Model file for the job. Use its own axes, mm. Face numbers are marked on the shaded views. A direction names the side the tool comes from. Coordinates: 2 decimals unless noted, no trailing zeros. Order: outer loops, then holes, each group sorted by start corner. A loop starts at its lowest first (then second) coordinate and runs counter-clockwise, first axis right, second up. Notation, with made-up numbers: (-9.5, -1) -> (34.5, -1) arc R16 cw to (34.5, 9) -> close; hole circle Ø10 at (-14.5, -2). An arc over 180 degrees is marked (long way). Write item = value, one per line. Start each with the question number.
Q1. Cut at A-A, the plane y = 34. List the corners of the cut face in (x, z), plus the area to 3 significant figures.
Q2. Cut at C-C, the plane x = -14.25. Give the number of separate pieces and of enclosed holes in the cut face, plus the area to 3 significant figures.
Q3. Mould opens along X. For the marked faces 1, 2 and 3 say: +X half, -X half, draft (parallel to the pull), parting line (faces both ways), or undercut.
Q4. Flat gauge pins, fed straight in: pin 1 (6 mm diameter, centred on x = -1, y = 22.5, fed in from -Z); pin 2 (2.5 mm diameter, centred on x = 1, z = 11, fed in from +Y); pin 3 (1.2 mm diameter, centred on x = 2.5, z = 11, fed in from +Y); pin 4 (5 mm diameter, centred on x = 2.5, z = 8, fed in from -Y). Where does each tip first touch, or does it go through?
Q5. 3-axis set-ups, long thin cutter, end or side, ignore diameter. For the marked faces 4, 5, 6 and 7: which of +Z, -Z, +X, -X, +Y, -Y reach the whole face in a straight line?
Q6. Cut at B-B, the plane z = -15. List the corners of the cut face in (x, y), plus the area to 3 significant figures.
Q7. Wall check: line 1 (X direction, y = 37.05, z = 0); line 2 (X direction, y = 35, z = 0); line 3 (Z direction, x = 14.25, y = 1.5) (3 decimals). Give the ranges that are in metal, low to high. Write a range as from..to.
from build123d import *

# Parameters (mm, degrees)
SKETCH1_W               = 48
SKETCH1_H               = 20
BOSS_EXTRUDE1_DEPTH     = 14.5
FILLET1_R               = 1
SKETCH2_R               = 9.5
BOSS_EXTRUDE2_DEPTH     = 25
SKETCH3_W               = 10.545517328
SKETCH3_H               = 9.5
BOSS_EXTRUDE3_DEPTH     = 22
FILLET2_R               = 5
SKETCH4_R               = 1
CUT_EXTRUDE1_DEPTH      = 5
SKETCH5_R               = 7.25
CUT_EXTRUDE2_DEPTH      = 13
SKETCH6_W               = 0.5
SKETCH6_H               = 2
SKETCH8_R               = 7.25
CUT_EXTRUDE3_DEPTH      = 3
SKETCH9_W               = 0.5
SKETCH9_H               = 2
SKETCH11_W              = 9
SKETCH11_H              = 3.5
BOSS_EXTRUDE4_DEPTH     = 3
SKETCH12_W              = 6.5
SKETCH12_H              = 0.5
BOSS_EXTRUDE5_DEPTH     = 0.8
SKETCH13_W              = 9
SKETCH13_H              = 0.25
BOSS_EXTRUDE6_DEPTH     = 1
SKETCH14_W              = 12
SKETCH14_H              = 1.5
BOSS_EXTRUDE7_DEPTH     = 0.8
CUT_EXTRUDE4_DEPTH      = 5
SKETCH16_W              = 7.75
SKETCH16_H              = 7.75
SKETCH16_R              = 2
BOSS_EXTRUDE8_DEPTH     = 2.5
MIRROR4_COPY_1_SKETCH_W = 7.75
MIRROR4_COPY_1_SKETCH_H = 7.75
MIRROR4_COPY_1_SKETCH_R = 2
MIRROR4_COPY_1_DEPTH    = 2.5
FILLET3_RADIUS          = 3.875
FILLET3_LENGTH          = 2.5
FILLET5_RADIUS          = 3.875
FILLET5_LENGTH          = 2.5
FILLET6_RADIUS          = 3.875
FILLET6_LENGTH          = 2.5
FILLET7_RADIUS          = 3.875
FILLET7_LENGTH          = 2.5
FILLET4_R               = 3
SKETCH17_W              = 7
SKETCH17_H              = 1.5
CUT_EXTRUDE5_DEPTH      = 3
SKETCH18_W              = 0.1
SKETCH18_H              = 1.5
BOSS_EXTRUDE9_DEPTH     = 3
SKETCH19_R              = 0.375
BOSS_EXTRUDE10_DEPTH    = 10


with BuildPart() as part:
    # Sketch1 → Boss-Extrude1 (new body)
    with BuildSketch(Plane(origin=(0, 0, 0), x_dir=(1, 0, 0), z_dir=(0, 1, 0))):
        Rectangle(SKETCH1_W, SKETCH1_H)
    extrude(amount=BOSS_EXTRUDE1_DEPTH)

    # Fillet1
    fillet1_edges = [part.edges().sort_by_distance(p)[0] for p in [
        (-24, 7.25, -10),
        (24, 7.25, -10),
        (24, 7.25, 10),
        (-24, 7.25, 10),
    ]]
    fillet(fillet1_edges, radius=FILLET1_R)

    # Sketch2 → Boss-Extrude2 (add)
    with BuildSketch(Plane(origin=(0, 14.5, 0), x_dir=(1, 0, 0), z_dir=(0, 1, 0))):
        with Locations(Location((-13.5, 0, 0), (0, 0, 270))):
            Circle(SKETCH2_R)
        with Locations(Location((13.5, 0, 0), (0, 0, 90))):
            Circle(SKETCH2_R)
    extrude(amount=BOSS_EXTRUDE2_DEPTH)

    # Sketch3 → Boss-Extrude3 (add)
    with BuildSketch(Plane(origin=(0, 14.5, 0), x_dir=(1, 0, 0), z_dir=(0, 1, 0))):
        Rectangle(SKETCH3_W, SKETCH3_H)
    extrude(amount=BOSS_EXTRUDE3_DEPTH)

    # Fillet2
    fillet2_edges = [part.edges().sort_by_distance(p)[0] for p in [
        (-5.272758664, 25.5, -4.75),
        (-5.272758664, 25.5, 4.75),
        (5.272758664, 25.5, 4.75),
        (5.272758664, 25.5, -4.75),
    ]]
    fillet(fillet2_edges, radius=FILLET2_R)

    # Sketch4 → Cut-Extrude1 (cut)
    with BuildSketch(Plane(origin=(0, 36.5, 0), x_dir=(1, 0, 0), z_dir=(0, 1, 0))):
        with Locations(Location((0, 0, 0), (0, 0, 270))):
            Circle(SKETCH4_R)
    extrude(amount=-CUT_EXTRUDE1_DEPTH, mode=Mode.SUBTRACT)

    # Sketch5 → Cut-Extrude2 (cut)
    with BuildSketch(Plane(origin=(0, 39.5, 0), x_dir=(1, 0, 0), z_dir=(0, 1, 0))):
        with Locations(Location((-13.5, 0, 0), (0, 0, 270))):
            Circle(SKETCH5_R)
    extrude(amount=-CUT_EXTRUDE2_DEPTH, mode=Mode.SUBTRACT)

    # Sketch6 → Revolve1 (revolve)
    with BuildSketch(Plane.XY, mode=Mode.PRIVATE) as revolve1_sk:
        with Locations((-20.5, 27.5)):
            Rectangle(SKETCH6_W, SKETCH6_H)
    revolve(revolve1_sk.sketch.rotate(Axis((-13.5, 39.5, 0), (0, -1, 0)), 270), axis=Axis((-13.5, 39.5, 0), (0, -1, 0)))

    # Sketch7 → Revolve2 (revolve)
    with BuildSketch(Plane.XY, mode=Mode.PRIVATE) as revolve2_sk:
        with BuildLine():
            Line((-20.25, 26.5), (-13.5, 26.5))
            Line((-13.5, 26.5), (-13.5, 28.5))
            add(Edge.make_bspline(
                [(-13.5, 28.5), (-20.25, 28.5), (-20.25, 26.5)],
                knots=[4.71238898, 4.71238898, 4.71238898, 6.283185307, 6.283185307, 6.283185307], degree=2, weights=[1, 0.707106781, 1]))
        make_face()
    revolve(revolve2_sk.sketch.rotate(Axis((-13.5, 26.5, 0), (0, 1, 0)), 222.253636979), axis=Axis((-13.5, 26.5, 0), (0, 1, 0)))

    # Sketch8 → Cut-Extrude3 (cut)
    with BuildSketch(Plane(origin=(0, 39.5, 0), x_dir=(1, 0, 0), z_dir=(0, 1, 0))):
        with Locations(Location((13.5, 0, 0), (0, 0, 270))):
            Circle(SKETCH8_R)
    extrude(amount=-CUT_EXTRUDE3_DEPTH, mode=Mode.SUBTRACT)

    # Sketch9 → Revolve3 (revolve)
    with BuildSketch(Plane.XY, mode=Mode.PRIVATE) as revolve3_sk:
        with Locations((20.5, 37.5)):
            Rectangle(SKETCH9_W, SKETCH9_H)
    revolve(revolve3_sk.sketch.rotate(Axis((13.5, 36.5, 0), (0, 1, 0)), 270), axis=Axis((13.5, 36.5, 0), (0, 1, 0)))

    # Sketch11 → Boss-Extrude4 (add)
    with BuildSketch(Plane.XY.offset(10)):
        with Locations((1.5, 9.25)):
            Rectangle(SKETCH11_W, SKETCH11_H)
    extrude(amount=BOSS_EXTRUDE4_DEPTH)

    # Sketch12 → Boss-Extrude5 (add)
    with BuildSketch(Plane.XY.offset(13)):
        with Locations((1.5, 11.25)):
            Rectangle(SKETCH12_W, SKETCH12_H)
    extrude(amount=-BOSS_EXTRUDE5_DEPTH)

    # Sketch13 → Boss-Extrude6 (add)
    with BuildSketch(Plane.XY.offset(13)):
        with Locations((1.5, 7.375)):
            Rectangle(SKETCH13_W, SKETCH13_H)
    extrude(amount=-BOSS_EXTRUDE6_DEPTH)

    # Sketch14 → Boss-Extrude7 (add)
    with BuildSketch(Plane.XY.offset(10)):
        with Locations((1.5, 6.25)):
            Rectangle(SKETCH14_W, SKETCH14_H)
    extrude(amount=BOSS_EXTRUDE7_DEPTH)

    # Sketch15 → Cut-Extrude4 (cut)
    with BuildSketch(Plane.XY.offset(10)):
        Polygon((-4.5, 7), (-4.5, 13), (7.5, 13), (7.5, 7), (6.5, 7), (6.5, 11.5), (-3.5, 11.5), (-3.5, 7), align=None)
    extrude(amount=-CUT_EXTRUDE4_DEPTH, mode=Mode.SUBTRACT)

    # Sketch16 → Boss-Extrude8 (add)
    with BuildSketch(Plane.XZ):
        with Locations((-14.25, 13.875)):
            Rectangle(SKETCH16_W, SKETCH16_H)
        with Locations(Location((-14.25, 13.875, 0), (0, 0, 270))):
            Circle(SKETCH16_R, mode=Mode.SUBTRACT)
    boss_extrude8 = extrude(amount=-BOSS_EXTRUDE8_DEPTH)

    # Mirror3: Boss-Extrude8 across plane
    add(boss_extrude8.mirror(Plane.XY))

    # Mirror4: Boss-Extrude8 across plane
    add(boss_extrude8.mirror(Plane(origin=(0, 0, 0), x_dir=(0, 0, 1), z_dir=(1, 0, 0))))

    # Mirror4 copy 1 sketch → Mirror4 copy 1 (add)
    with BuildSketch(Plane(origin=(0, 0, 0), x_dir=(-1, 0, 0), z_dir=(0, -1, 0))):
        with Locations((-14.25, 13.875)):
            Rectangle(MIRROR4_COPY_1_SKETCH_W, MIRROR4_COPY_1_SKETCH_H)
        with Locations(Location((-14.25, 13.875, 0), (0, 0, 270))):
            Circle(MIRROR4_COPY_1_SKETCH_R, mode=Mode.SUBTRACT)
    extrude(amount=-MIRROR4_COPY_1_DEPTH)

    # Fillet3: full round fillet: the end face becomes a half cylinder, R = half its width
    fillet3_face = Plane((-14.25, 1.25, 17.75), x_dir=(0, -1, 0), z_dir=(0, 0, 1))  # on the end face: x along it, z out of the body
    fillet3_slab = fillet3_face.offset(-FILLET3_RADIUS / 2) * Box(FILLET3_LENGTH, 2 * FILLET3_RADIUS, FILLET3_RADIUS, mode=Mode.PRIVATE)  # the body's end, R deep
    fillet3_round = Plane((-14.25, 1.25, 13.875), x_dir=(0, 0, 1), z_dir=(0, -1, 0)) * Cylinder(FILLET3_RADIUS, FILLET3_LENGTH, mode=Mode.PRIVATE)  # its axis R under the face
    add(fillet3_slab - fillet3_round, mode=Mode.SUBTRACT)

    # Fillet5: full round fillet: the end face becomes a half cylinder, R = half its width
    fillet5_face = Plane((14.25, 1.25, 17.75), x_dir=(0, 1, 0), z_dir=(0, 0, 1))  # on the end face: x along it, z out of the body
    fillet5_slab = fillet5_face.offset(-FILLET5_RADIUS / 2) * Box(FILLET5_LENGTH, 2 * FILLET5_RADIUS, FILLET5_RADIUS, mode=Mode.PRIVATE)  # the body's end, R deep
    fillet5_round = Plane((14.25, 1.25, 13.875), x_dir=(0, 0, 1), z_dir=(0, 1, 0)) * Cylinder(FILLET5_RADIUS, FILLET5_LENGTH, mode=Mode.PRIVATE)  # its axis R under the face
    add(fillet5_slab - fillet5_round, mode=Mode.SUBTRACT)

    # Fillet6: full round fillet: the end face becomes a half cylinder, R = half its width
    fillet6_face = Plane((-14.25, 1.25, -17.75), x_dir=(0, 1, 0), z_dir=(0, 0, -1))  # on the end face: x along it, z out of the body
    fillet6_slab = fillet6_face.offset(-FILLET6_RADIUS / 2) * Box(FILLET6_LENGTH, 2 * FILLET6_RADIUS, FILLET6_RADIUS, mode=Mode.PRIVATE)  # the body's end, R deep
    fillet6_round = Plane((-14.25, 1.25, -13.875), x_dir=(0, 0, -1), z_dir=(0, 1, 0)) * Cylinder(FILLET6_RADIUS, FILLET6_LENGTH, mode=Mode.PRIVATE)  # its axis R under the face
    add(fillet6_slab - fillet6_round, mode=Mode.SUBTRACT)

    # Fillet7: full round fillet: the end face becomes a half cylinder, R = half its width
    fillet7_face = Plane((14.25, 1.25, -17.75), x_dir=(0, -1, 0), z_dir=(0, 0, -1))  # on the end face: x along it, z out of the body
    fillet7_slab = fillet7_face.offset(-FILLET7_RADIUS / 2) * Box(FILLET7_LENGTH, 2 * FILLET7_RADIUS, FILLET7_RADIUS, mode=Mode.PRIVATE)  # the body's end, R deep
    fillet7_round = Plane((14.25, 1.25, -13.875), x_dir=(0, 0, -1), z_dir=(0, -1, 0)) * Cylinder(FILLET7_RADIUS, FILLET7_LENGTH, mode=Mode.PRIVATE)  # its axis R under the face
    add(fillet7_slab - fillet7_round, mode=Mode.SUBTRACT)

    # Fillet4
    fillet4_edges = [part.edges().sort_by_distance(p)[0] for p in [
        (-18.125, 1.25, 10),
        (-10.375, 1.25, 10),
        (-18.125, 1.25, -10),
        (-10.375, 1.25, -10),
        (18.125, 1.25, 10),
        (10.375, 1.25, 10),
        (18.125, 1.25, -10),
        (10.375, 1.25, -10),
    ]]
    fillet(fillet4_edges, radius=FILLET4_R)

    # Sketch17 → Cut-Extrude5 (cut)
    with BuildSketch(Plane.XY.offset(13)):
        with Locations((1.5, 9)):
            Rectangle(SKETCH17_W, SKETCH17_H)
    extrude(amount=-CUT_EXTRUDE5_DEPTH, mode=Mode.SUBTRACT)

    # Sketch18 → Boss-Extrude9 (add)
    with BuildSketch(Plane.XY.offset(10)):
        with Locations((-0.833333333, 9)):
            Rectangle(SKETCH18_W, SKETCH18_H)
        with Locations((0.333333333, 9)):
            Rectangle(SKETCH18_W, SKETCH18_H)
        with Locations((1.5, 9)):
            Rectangle(SKETCH18_W, SKETCH18_H)
        with Locations((2.666666667, 9)):
            Rectangle(SKETCH18_W, SKETCH18_H)
        with Locations((3.833333333, 9)):
            Rectangle(SKETCH18_W, SKETCH18_H)
    extrude(amount=BOSS_EXTRUDE9_DEPTH)

    # Sketch19 → Boss-Extrude10 (add)
    with BuildSketch(Plane.XY.offset(10)):
        with Locations((-1.441666667, 9)):
            Circle(SKETCH19_R)
        with Locations((2.083333333, 9)):
            Circle(SKETCH19_R)
        with Locations((3.25, 9)):
            Circle(SKETCH19_R)
        with Locations((4.441666667, 9)):
            Circle(SKETCH19_R)
    extrude(amount=BOSS_EXTRUDE10_DEPTH)


solid = part.part
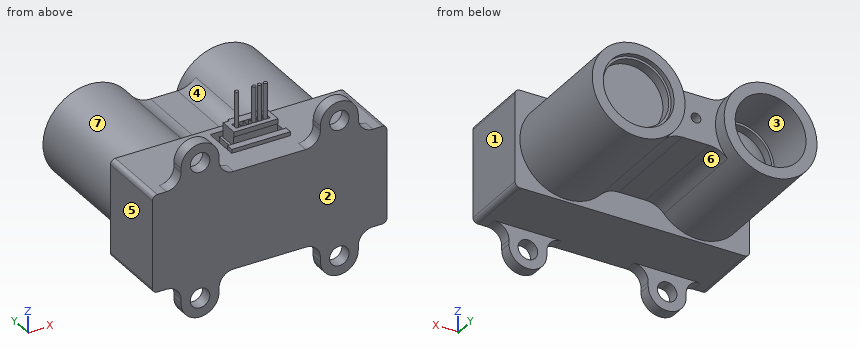
Here are the results:
q1.outline = (-6.47, -6.39) arc R5 cw to (-2.77, -4.75) -> (2.77, -4.75) arc R5 cw to (6.47, -6.39) arc R9.5 ccw (long way) to (6.47, 6.39) arc R5 cw to (2.77, 4.75) -> (-2.77, 4.75) arc R5 cw to (-6.47, 6.39) arc R9.5 ccw (long way) to start; hole circle Ø14.5 at (-13.5, 0); hole circle Ø2 at (0, 0)
q1.area = 486 mm²
q2.separate_pieces = 3
q2.enclosed_holes = 0
q2.area = 618 mm²
q3.face_1 = +X half
q3.face_2 = draft
q3.face_3 = undercut
q4.pin_1 = -4.9
q4.pin_2 = 14.5
q4.pin_3 = 11
q4.pin_4 = 0
q5.face_4 = +Z, +Y
q5.face_5 = +Z, -Z, -X, +Y, -Y
q5.face_6 = -Z, +Y
q5.face_7 = +Y
q6.outline = (-17.96, 0) -> (-15.9, 0) -> (-15.9, 2.5) -> (-17.96, 2.5) -> close; (-12.6, 0) -> (-10.54, 0) -> (-10.54, 2.5) -> (-12.6, 2.5) -> close; (10.54, 0) -> (12.6, 0) -> (12.6, 2.5) -> (10.54, 2.5) -> close; (15.9, 0) -> (17.96, 0) -> (17.96, 2.5) -> (15.9, 2.5) -> close
q6.area = 20.5 mm²
q7.line_1 = -23..-20.75, -6.25..-4, 4..6.75, 20.25..23
q7.line_2 = -23..-20.75, -6.25..-1, 1..23
q7.line_3 = -17.75..-15.875, -11.875..11.875, 15.875..17.75
